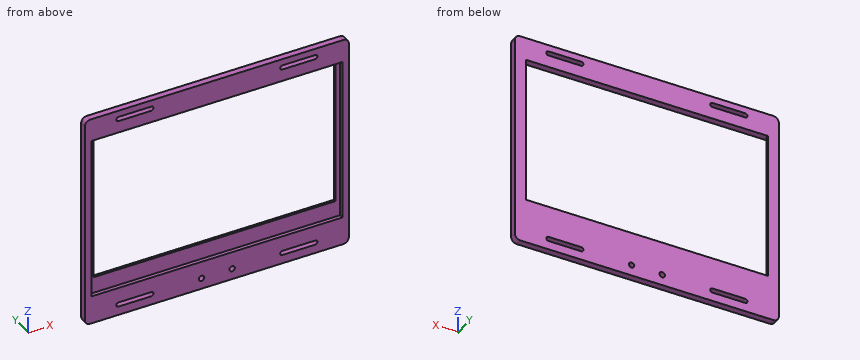
from build123d import *

# Parameters (mm, degrees)
SKETCH1_W               = 241.5
SKETCH1_H               = 197
SKETCH1_R               = 2.5
BOSS_EXTRUDE1_DEPTH     = 6
SKETCH1_5_W             = 229.5
SKETCH1_5_H             = 150
CUT_EXTRUDE1_DEPTH      = 3.7
FILLET1_R               = 5
CUT_EXTRUDE3_DEPTH      = 158.465083431
CUT_EXTRUDE3_DEPTH_BACK = 158.465083431


with BuildPart() as part:
    # Sketch1 → Boss-Extrude1 (new body)
    with BuildSketch(Plane(origin=(0, 0, 0), x_dir=(1, 0, 0), z_dir=(0, 1, 0))):
        with Locations((0, 2.5)):
            Rectangle(SKETCH1_W, SKETCH1_H)
        with BuildLine():
            ThreePointArc((90, 93), (92, 91), (90, 89))
            Line((90, 89), (60, 89))
            ThreePointArc((60, 89), (58, 91), (60, 93))
            Line((60, 93), (90, 93))
        make_face(mode=Mode.SUBTRACT)
        with BuildLine():
            ThreePointArc((-90, 89), (-92, 91), (-90, 93))
            Line((-90, 93), (-60, 93))
            ThreePointArc((-60, 93), (-58, 91), (-60, 89))
            Line((-60, 89), (-90, 89))
        make_face(mode=Mode.SUBTRACT)
        with Locations(Location((-14, 91, 0), (0, 0, 270))):
            Circle(SKETCH1_R, mode=Mode.SUBTRACT)
        with Locations(Location((14, 91, 0), (0, 0, 270))):
            Circle(SKETCH1_R, mode=Mode.SUBTRACT)
        with BuildLine():
            ThreePointArc((90, -86), (92, -88), (90, -90))
            Line((90, -90), (60, -90))
            ThreePointArc((60, -90), (58, -88), (60, -86))
            Line((60, -86), (90, -86))
        make_face(mode=Mode.SUBTRACT)
        with BuildLine():
            ThreePointArc((-90, -90), (-92, -88), (-90, -86))
            Line((-90, -86), (-60, -86))
            ThreePointArc((-60, -86), (-58, -88), (-60, -90))
            Line((-60, -90), (-90, -90))
        make_face(mode=Mode.SUBTRACT)
    extrude(amount=BOSS_EXTRUDE1_DEPTH)

    # Sketch1<5> → Cut-Extrude1 (cut)
    with BuildSketch(Plane(origin=(0, 0, 0), x_dir=(1, 0, 0), z_dir=(0, 1, 0))):
        Rectangle(SKETCH1_5_W, SKETCH1_5_H)
    extrude(amount=CUT_EXTRUDE1_DEPTH, mode=Mode.SUBTRACT)

    # Fillet1
    fillet1_edges = [part.edges().sort_by_distance(p)[0] for p in [
        (-120.75, 3, -101),
        (120.75, 3, -101),
        (-120.75, 3, 96),
        (120.75, 3, 96),
    ]]
    fillet(fillet1_edges, radius=FILLET1_R)

    # Sketch2 → Cut-Extrude3 (cut, two sides: drawn at the far end of the back side and taken through both)
    with BuildSketch(Plane.XZ.offset(-3.7).offset(-CUT_EXTRUDE3_DEPTH_BACK)):
        Polygon((94.75, -60), (110.75, -60), (110.75, 75), (94.75, 75), (-94.75, 75), (-110.75, 75), (-110.75, -60), align=None)
    extrude(amount=CUT_EXTRUDE3_DEPTH + CUT_EXTRUDE3_DEPTH_BACK, mode=Mode.SUBTRACT)


solid = part.part
The listing builds one solid part. Answer for the finished solid, in the listing's coordinates (mm). Give positions to 0.01 mm unless a question says otherwise; leave off trailing zeros. Order: outer loops, then holes, each group sorted by start corner. A loop starts at its lowest first (then second) coordinate and runs counter-clockwise, first axis right, second up. Notation, with made-up numbers: (54.5, 15.5) - (111.5, 15.5) arc R26 cw to (111.5, 39.5) - close; hole circle Ø6 at (-6, 73). An arc over 180 degrees is marked (long way). Use one line per item in the form item = value.
1) Find section C-C on y = 1.85. Give the number of separate pieces and of enclosed holes in the cut face, and give its area (3 significant figures).
Verdict:
separate_pieces = 1
enclosed_holes = 7
area = 12,600 mm^2
2) This flat-tipped pin is pushed along its axis until it touches: pin 1 (8 mm diameter, centred on x = 14, z = -91, fed in from +Y). Where does it stop, or does it pass through?
Verdict:
pin_1 = 6
3) Find section B-B on x = 14. Determine the outline of the cut face in (y, z).
Verdict:
outline = (0, -101) - (6, -101) - (6, -93.5) - (0, -93.5) - close; (0, -88.5) - (6, -88.5) - (6, -60) - (3.7, -60) - (3.7, -75) - (0, -75) - close; (0, 75) - (6, 75) - (6, 96) - (0, 96) - close
4) Find section A-A on z = -13. Determine the outline of the cut face in (x, y).
Verdict:
outline = (-120.75, 0) - (-114.75, 0) - (-114.75, 3.7) - (-110.75, 3.7) - (-110.75, 6) - (-120.75, 6) - close; (110.75, 3.7) - (114.75, 3.7) - (114.75, 0) - (120.75, 0) - (120.75, 6) - (110.75, 6) - close
5) Consider probe 1 along X at (y, z) = (4.25, -91); probe 2 along Z at (x, y) = (-44, 0.85); probe 3 along Z at (x, y) = (47, 5.6). Determine where each line is inside the solid, lowest interval first. Write a range as [from, to].
Verdict:
probe_1 = [-120.75, -92], [-58, -16.5], [-11.5, 11.5], [16.5, 58], [92, 120.75]
probe_2 = [-101, -75], [75, 96]
probe_3 = [-101, -60], [75, 96]
